from build123d import *

# Parameters (mm, degrees)
SKETCH1_R           = 17.6
BOSS_EXTRUDE1_DEPTH = 21.8
SKETCH2_R           = 4.5
BOSS_EXTRUDE2_DEPTH = 2.7
SKETCH3_R           = 1.5
BOSS_EXTRUDE3_DEPTH = 6.3
BOSS_EXTRUDE4_START = 2.7
SKETCH4_R           = 4.5
BOSS_EXTRUDE4_DEPTH = 2.7
BOSS_EXTRUDE5_START = 2.5
SKETCH5_R           = 1.5
BOSS_EXTRUDE5_DEPTH = 2.5
SKETCH6_R           = 1.75
CUT_EXTRUDE1_DEPTH  = 2.5
CHAMFER1_SIZE       = 0.25
CHAMFER2_SIZE       = 0.3
FILLET1_R           = 1
CHAMFER3_SIZE       = 0.3


with BuildPart() as part:
    # Sketch1 → Boss-Extrude1 (new body)
    with BuildSketch(Plane.XY):
        Circle(SKETCH1_R)
    extrude(amount=BOSS_EXTRUDE1_DEPTH)

    # Sketch2 → Boss-Extrude2 (add)
    with BuildSketch(Plane.XY.offset(21.8)):
        with Locations(Location((0, 0, 0), (0, 0, 180))):
            Circle(SKETCH2_R)
    extrude(amount=BOSS_EXTRUDE2_DEPTH)

    # Sketch3 → Boss-Extrude3 (add)
    with BuildSketch(Plane.XY.offset(24.5)):
        Circle(SKETCH3_R)
    extrude(amount=BOSS_EXTRUDE3_DEPTH)

    # Sketch4 → Boss-Extrude4 (add)
    with BuildSketch(Plane(origin=(0, 0, 0), x_dir=(-1, 0, 0), z_dir=(0, 0, -1)).offset(BOSS_EXTRUDE4_START)):
        Circle(SKETCH4_R)
    extrude(amount=-BOSS_EXTRUDE4_DEPTH)

    # Sketch5 → Boss-Extrude5 (add)
    with BuildSketch(Plane(origin=(0, 0, -2.7), x_dir=(-1, 0, 0), z_dir=(0, 0, -1)).offset(BOSS_EXTRUDE5_START)):
        with Locations(Location((0, 0, 0), (0, 0, 180))):
            Circle(SKETCH5_R)
    extrude(amount=-BOSS_EXTRUDE5_DEPTH)

    # Sketch6 → Cut-Extrude1 (cut)
    with BuildSketch(Plane.XY.offset(21.8)):
        with Locations((0, 12.5)):
            Circle(SKETCH6_R)
        with Locations((12.5, 0)):
            Circle(SKETCH6_R)
        with Locations((0, -12.5)):
            Circle(SKETCH6_R)
        with Locations((-12.5, 0)):
            Circle(SKETCH6_R)
    extrude(amount=-CUT_EXTRUDE1_DEPTH, mode=Mode.SUBTRACT)

    # Chamfer1
    chamfer1_edges = [part.edges().sort_by_distance(p)[0] for p in [
        (-1.75, 12.5, 21.8),
        (10.75, 0, 21.8),
        (-1.75, -12.5, 21.8),
        (-14.25, 0, 21.8),
    ]]
    chamfer(chamfer1_edges, length=CHAMFER1_SIZE)

    # Chamfer2
    chamfer2_edges = [part.edges().sort_by_distance(p)[0] for p in [
        (4.5, 0, -2.7),
        (4.5, 0, 24.5),
    ]]
    chamfer(chamfer2_edges, length=CHAMFER2_SIZE)

    # Fillet1
    fillet1_edges = [part.edges().sort_by_distance(p)[0] for p in [
        (-17.6, 0, 21.8),
    ]]
    fillet(fillet1_edges, radius=FILLET1_R)

    # Chamfer3
    chamfer3_edges = [part.edges().sort_by_distance(p)[0] for p in [
        (-1.5, 0, 30.8),
        (-1.5, 0, -5.2),
    ]]
    chamfer(chamfer3_edges, length=CHAMFER3_SIZE)


solid = part.part
Geometry: final body of the model. Coordinates: model frame, mm. A direction names the side the tool comes from. Coordinates: 2 decimals unless noted, no trailing zeros. Return JSON: item names as keys, results as strings.
Item 1: Line query: L1, parallel to Y at x = 0, z = 20.8; L2, parallel to Z at x = -12.5, y = -1; L3, parallel to Z at x = 8, y = 11. Output: solid intervals per line, ascending.
Completed:
{"L1": "y = -17.6 to -14.25, -10.75 to 10.75, 14.25 to 17.6", "L2": "z = 0 to 19.3", "L3": "z = 0 to 21.8"}
Item 2: Pull-direction query (X, two-part tool) for faces 4 (the face through (0, 0, 30.8)), 5 (the face through (-13, 0, 19.3)), 6 (the face through (-1.5, 0.07, 27.46)); classes: +X half, -X half, draft (parallel to the pull), parting line (faces both ways), or undercut.
Completed:
{"face 4": "draft", "face 5": "undercut", "face 6": "parting line"}
Item 3: Reachability of faces 1 (the face through (1.43, -0.45, -3.82)), 2 (the face through (16.787, 5.287, 10.254)), 3 (the face through (0, 13, 19.3)) from +Z, -Z, +X, -X, +Y, -Y: full face, straight path, thin tool, end or side. Return the list, or none.
Completed:
{"face 1": "-Z", "face 2": "+Z, -Z", "face 3": "+Z"}
Item 4: Pin query (flat end, axial travel): pin 1 Ø4 at (x, y) = (9.5, 9) entering from +Z; pin 2 Ø6.5 at (x, y) = (-2, -1) entering from -Z; pin 3 Ø3 at (x, y) = (12.5, 0) entering from +Z; pin 4 Ø12 at (x, y) = (-11, 10) entering from -Z. Return the tip coordinate at first contact, or that it passes through.
Completed:
{"pin 1": "stops at z = 21.8", "pin 2": "stops at z = -5.2", "pin 3": "stops at z = 19.3", "pin 4": "stops at z = 0"}
